from build123d import *

# Parameters (mm, degrees)
ESQUISSE1_R                        = 1.7
BOSS_EXTRU_1_DEPTH                 = 4
CONG_1_R                           = 3
R_P_TITION_CIRCULAIRE1_COUNT       = 4
CONG_1_OF_R_P_TITION_CIRCULAIRE1_R = 3
CHANFREIN1_SIZE                    = 1.05
BOSS_EXTRU_2_REACH                 = 56.194
ESQUISSE2_R                        = 2.4
CONG_2_R                           = 3
ESQUISSE2_2_R                      = 2.4
BOSS_EXTRU_3_DEPTH                 = 1
M3_CLEARANCE_HOLE1_D               = 3.4
CHANFREIN2_SIZE                    = 0.5


with BuildPart() as part:
    # Sketch1 → Revolve1 (revolve)
    with BuildSketch(Plane.XY, mode=Mode.PRIVATE) as revolve1_sk:
        Polygon((6.5, 0), (27, 0), (27, 3), (29, 3), (29, 7), (4.25, 7), (4.25, 5), (5.5, 5), (5.5, 1), align=None)
    revolve(revolve1_sk.sketch.rotate(Axis((0, 16.318563478, 0), (0, -1, 0)), 90), axis=Axis((0, 16.318563478, 0), (0, -1, 0)))

    # Esquisse1 → Boss.-Extru.1 (add)
    with BuildSketch(Plane(origin=(0, 7, 0), x_dir=(1, 0, 0), z_dir=(0, 1, 0))):
        with BuildLine():
            Line((-5, 33), (-5, 28.565713714))
            ThreePointArc((-5, 28.565713714), (0, 29), (5, 28.565713714))
            Line((5, 28.565713714), (5, 33))
            ThreePointArc((5, 33), (0, 38), (-5, 33))
        make_face()
        with Locations(Location((0, 33, 0), (0, 0, 270))):
            Circle(ESQUISSE1_R, mode=Mode.SUBTRACT)
    boss_extru_1 = extrude(amount=-BOSS_EXTRU_1_DEPTH)

    # Congé1
    cong_1_edges = [part.edges().sort_by_distance(p)[0] for p in [
        (-5, 5, -28.565713714),
        (5, 5, -28.565713714),
    ]]
    fillet(cong_1_edges, radius=CONG_1_R)

    # Répétition circulaire1: Boss.-Extru.1 ×4 about axis
    r_p_tition_circulaire1_axis = Axis((0, 0, 0), (0, 1, 0))
    for i in range(1, R_P_TITION_CIRCULAIRE1_COUNT):
        add(boss_extru_1.rotate(r_p_tition_circulaire1_axis, i * 360 / R_P_TITION_CIRCULAIRE1_COUNT))

    # Congé1 of Répétition circulaire1
    cong_1_of_r_p_tition_circulaire1_edges = [part.edges().sort_by_distance(p)[0] for p in [
        (-28.565713714, 5, 5),
        (-28.565713714, 5, -5),
        (5, 5, 28.565713714),
        (-5, 5, 28.565713714),
        (28.565713714, 5, -5),
        (28.565713714, 5, 5),
    ]]
    fillet(cong_1_of_r_p_tition_circulaire1_edges, radius=CONG_1_OF_R_P_TITION_CIRCULAIRE1_R)

    # Chanfrein1
    chanfrein1_edges = [part.edges().sort_by_distance(p)[0] for p in [
        (0, 7, -34.7),
        (34.7, 7, 0),
        (0, 7, 34.7),
        (-34.7, 7, 0),
    ]]
    chamfer(chanfrein1_edges, length=CHANFREIN1_SIZE)

    # Boss.-Extru.2: up to this face of the body (flat: up to its plane)
    boss_extru_2_end = Plane(part.part.faces().sort_by_distance((0, 0, -7.263675324))[0])
    # Esquisse2 → Boss.-Extru.2 (add, up to the picked face)
    with BuildSketch(Plane(origin=(0, 7, 0), x_dir=(1, 0, 0), z_dir=(0, 1, 0)), mode=Mode.PRIVATE) as boss_extru_2_sk1:
        with BuildLine():
            Line((-12.169872981, 31.078838325), (-8.936372142, 25.478250586))
            ThreePointArc((-8.936372142, 25.478250586), (-13.5, 23.382685902), (-17.59662618, 20.478250586))
            Line((-17.59662618, 20.478250586), (-20.830127019, 26.078838325))
            ThreePointArc((-20.830127019, 26.078838325), (-19, 32.908965344), (-12.169872981, 31.078838325))
        make_face()
        with Locations(Location((-16.5, 28.578838325, 0), (0, 0, 270))):
            Circle(ESQUISSE2_R, mode=Mode.SUBTRACT)
    boss_extru_2_tool1 = split(extrude(boss_extru_2_sk1.sketch, amount=-BOSS_EXTRU_2_REACH, mode=Mode.PRIVATE), bisect_by=boss_extru_2_end, keep=Keep.BOTH, mode=Mode.PRIVATE)
    # Esquisse2 → Boss.-Extru.2 (add, up to the picked face)
    with BuildSketch(Plane(origin=(0, 7, 0), x_dir=(1, 0, 0), z_dir=(0, 1, 0)), mode=Mode.PRIVATE) as boss_extru_2_sk2:
        with BuildLine():
            Line((31.078838325, 12.169872981), (25.478250586, 8.936372142))
            ThreePointArc((25.478250586, 8.936372142), (23.382685902, 13.5), (20.478250586, 17.59662618))
            Line((20.478250586, 17.59662618), (26.078838325, 20.830127019))
            ThreePointArc((26.078838325, 20.830127019), (32.908965344, 19), (31.078838325, 12.169872981))
        make_face()
        with Locations(Location((28.578838325, 16.5, 0), (0, 0, 270))):
            Circle(ESQUISSE2_R, mode=Mode.SUBTRACT)
    boss_extru_2_tool2 = split(extrude(boss_extru_2_sk2.sketch, amount=-BOSS_EXTRU_2_REACH, mode=Mode.PRIVATE), bisect_by=boss_extru_2_end, keep=Keep.BOTH, mode=Mode.PRIVATE)
    # Esquisse2 → Boss.-Extru.2 (add, up to the picked face)
    with BuildSketch(Plane(origin=(0, 7, 0), x_dir=(1, 0, 0), z_dir=(0, 1, 0)), mode=Mode.PRIVATE) as boss_extru_2_sk3:
        with BuildLine():
            Line((20.830127019, -26.078838325), (17.59662618, -20.478250586))
            ThreePointArc((17.59662618, -20.478250586), (13.5, -23.382685902), (8.936372142, -25.478250586))
            Line((8.936372142, -25.478250586), (12.169872981, -31.078838325))
            ThreePointArc((12.169872981, -31.078838325), (19, -32.908965344), (20.830127019, -26.078838325))
        make_face()
        with Locations(Location((16.5, -28.578838325, 0), (0, 0, 270))):
            Circle(ESQUISSE2_R, mode=Mode.SUBTRACT)
    boss_extru_2_tool3 = split(extrude(boss_extru_2_sk3.sketch, amount=-BOSS_EXTRU_2_REACH, mode=Mode.PRIVATE), bisect_by=boss_extru_2_end, keep=Keep.BOTH, mode=Mode.PRIVATE)
    # Esquisse2 → Boss.-Extru.2 (add, up to the picked face)
    with BuildSketch(Plane(origin=(0, 7, 0), x_dir=(1, 0, 0), z_dir=(0, 1, 0)), mode=Mode.PRIVATE) as boss_extru_2_sk4:
        with BuildLine():
            Line((-26.078838325, -20.830127019), (-20.478250586, -17.59662618))
            ThreePointArc((-20.478250586, -17.59662618), (-23.382685902, -13.5), (-25.478250586, -8.936372142))
            Line((-25.478250586, -8.936372142), (-31.078838325, -12.169872981))
            ThreePointArc((-31.078838325, -12.169872981), (-32.908965344, -19), (-26.078838325, -20.830127019))
        make_face()
        with Locations(Location((-28.578838325, -16.5, 0), (0, 0, 270))):
            Circle(ESQUISSE2_R, mode=Mode.SUBTRACT)
    boss_extru_2_tool4 = split(extrude(boss_extru_2_sk4.sketch, amount=-BOSS_EXTRU_2_REACH, mode=Mode.PRIVATE), bisect_by=boss_extru_2_end, keep=Keep.BOTH, mode=Mode.PRIVATE)
    add(boss_extru_2_tool1.solids().sort_by(Axis((-19.056182, 7, -23.369301), (0, -1, 0)))[0])
    add(boss_extru_2_tool2.solids().sort_by(Axis((32.75177, 7, -18.909243), (0, -1, 0)))[0])
    add(boss_extru_2_tool3.solids().sort_by(Axis((10.710318, 7, 28.187788), (0, -1, 0)))[0])
    add(boss_extru_2_tool4.solids().sort_by(Axis((-23.539881, 7, 13.590757), (0, -1, 0)))[0])

    # Congé2
    cong_2_edges = [part.edges().sort_by_distance(p)[0] for p in [
        (-22.238633754, 5, 18.612983876),
        (-27.238633754, 5, 9.952729838),
        (-18.612983876, 5, -22.238633754),
        (-9.952729838, 5, -27.238633754),
        (22.238633754, 5, -18.612983876),
        (27.238633754, 5, -9.952729838),
        (18.612983876, 5, 22.238633754),
        (9.952729838, 5, 27.238633754),
    ]]
    fillet(cong_2_edges, radius=CONG_2_R)

    # Esquisse2<2> → Boss.-Extru.3 (add)
    with BuildSketch(Plane(origin=(0, 7, 0), x_dir=(1, 0, 0), z_dir=(0, 1, 0))):
        with Locations(Location((16.5, -28.578838325, 0), (0, 0, 270))):
            Circle(ESQUISSE2_2_R)
        with Locations(Location((28.578838325, 16.5, 0), (0, 0, 270))):
            Circle(ESQUISSE2_2_R)
        with Locations(Location((-16.5, 28.578838325, 0), (0, 0, 270))):
            Circle(ESQUISSE2_2_R)
        with Locations(Location((-28.578838325, -16.5, 0), (0, 0, 270))):
            Circle(ESQUISSE2_2_R)
    extrude(amount=-BOSS_EXTRU_3_DEPTH)

    # M3 Clearance Hole1 (through all)
    with Locations(Plane(origin=(0, 7, 0), x_dir=(1, 0, 0), z_dir=(0, 1, 0))):
        with Locations((16.5, -28.578838325), (28.578838325, 16.5), (-16.5, 28.578838325), (-28.578838325, -16.5)):
            Hole(M3_CLEARANCE_HOLE1_D / 2)

    # Chanfrein2
    chanfrein2_edges = [part.edges().sort_by_distance(p)[0] for p in [
        (-28.578838325, 0, 14.1),
        (-16.5, 0, -30.978838325),
        (28.578838325, 0, -18.9),
        (16.5, 0, 26.178838325),
    ]]
    chamfer(chanfrein2_edges, length=CHANFREIN2_SIZE)


solid = part.part
Build history of the part. All positions in model axes, mm. A direction names the side the tool comes from. Round coordinates to 2 decimals unless told otherwise and drop trailing zeros. Write each loop counter-clockwise with the first axis right and the second up, starting at its lowest first coordinate (ties: lowest second). Pieces come first, ordered by that corner, then holes. Notation, with made-up numbers: (-21, -14.75) - (3, -14.75) arc R18 ccw to (3, 2.25) - close; hole circle Ø2 at (44.5, -37.75). An arc over 180 degrees is marked (long way). One line per question, with ' | ' between items.
1. Band-saw the part on D-D, the plane z = 16.5. Write the cut outline in (x, y), and give its area (3 significant figures).
Results are:
outline: (-33.58, 0) - (-31.48, 0) - (-30.98, 0.5) - (-30.98, 6) - (-30.28, 6) - (-30.28, 7) - (-33.58, 7) - close; (-26.88, 6) - (-26.18, 6) - (-26.18, 0.5) - (-25.68, 0) - (21.37, 0) - (21.37, 3) - (23.85, 3) - (23.85, 7) - (-26.88, 7) - close | area: 362 mm^2
2. Mould opens along X. For faces 1 (the face through (-0.65, 4.5, -31.43)), 2 (the face through (26.138, 1.521, 6.769)), 3 (the face through (-25.17, 5.03, -14.4)) say: released by +X, released by -X, zero draft, split by the parting line, or undercut.
Results are:
face 1: undercut | face 2: released by +X | face 3: released by -X
3. Band-saw the part on A-A, the plane z = 0. Give the number of separate pieces and of enclosed holes in the cut face, and give its area (3 significant figures).
Results are:
separate pieces: 4 | enclosed holes: 0 | area: 364 mm^2
4. Drop flat-ended pins along their axis: pin 1 Ø2 at (x, z) = (28.58, -16.5) entering from -Y; pin 2 Ø2.5 at (x, z) = (17, 27.5) entering from -Y; pin 3 Ø4.5 at (x, z) = (0, 33) entering from +Y; pin 4 Ø1 at (y, z) = (5.5, -32) entering from -X. Give the stop position or say it passes through.
Results are:
pin 1: through | pin 2: y = 0.46 | pin 3: y = 6.5 | pin 4: x = -20.56
5. Drill centre lines: line 1 along X through (y, z) = (2.4, 0); line 2 along X through (y, z) = (4.7, -33). Where is each one in solid material? Low to high. Write a range as from..to.
Results are:
line 1: -27..-5.5, 5.5..27 | line 2: -18.84..-14.16, -5..-1.7, 1.7..5
6. Tool access for faces 4 (the face through (5.37, 2.97, -1.19)), 5 (the face through (-26.138, 1.521, -6.769)), 6 (the face through (29.12, 4.97, -5.65)), 7 (the face through (0, 0, -7)), 8 (the face through (-10.935, 2.771, -28.94)): list every direction of +Z, -Z, +X, -X, +Y, -Y with a clear straight run to the whole face (end or side of a thin tool).
Results are:
face 4: -Y | face 5: -X, -Y | face 6: +X, +Y, -Y | face 7: +Z, -Z, +X, -X, -Y | face 8: -Z, -Y
7. Band-saw the part on C-C, the plane x = -16.5. Write the cut outline in (y, z).
Results are:
outline: (0, -33.58) - (7, -33.58) - (7, -30.28) - (6, -30.28) - (6, -30.98) - (0.5, -30.98) - (0, -31.48) - close; (0, -25.68) - (0.5, -26.18) - (6, -26.18) - (6, -26.88) - (7, -26.88) - (7, 23.85) - (3, 23.85) - (3, 21.37) - (0, 21.37) - close
